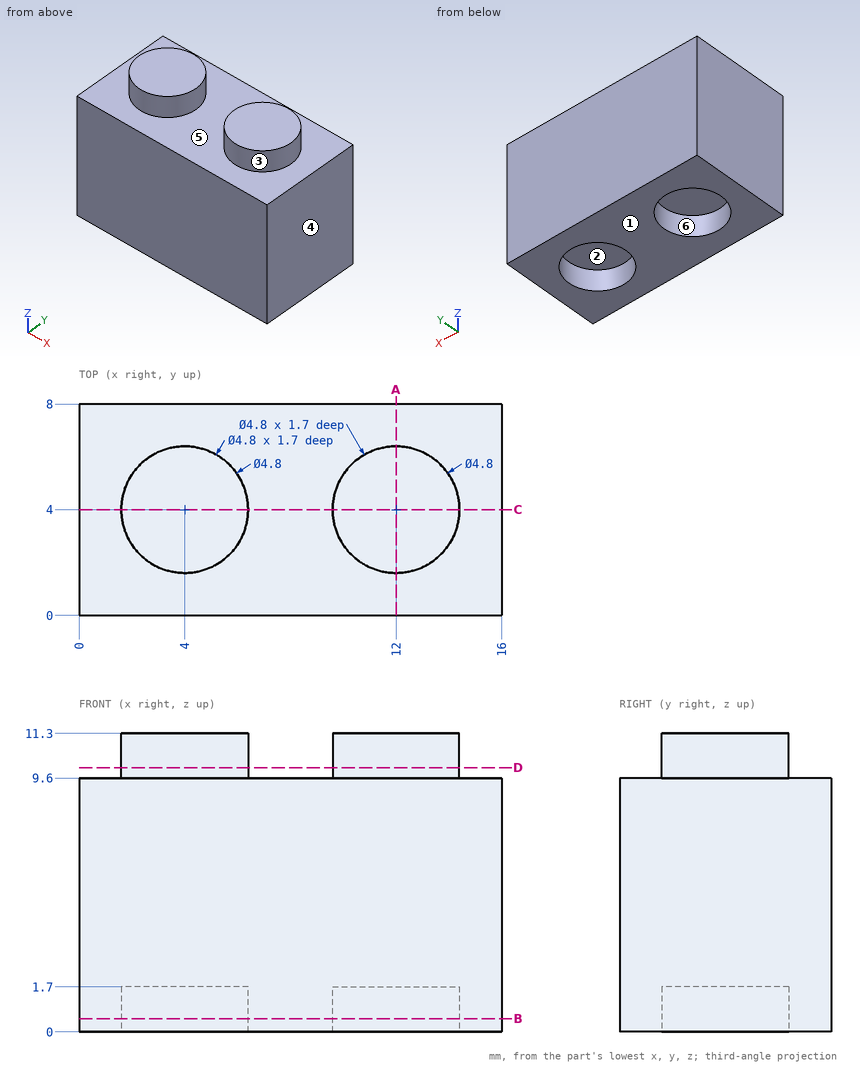
Could you check a few things on this drawing? It's one solid part, dimensions in mm from its lowest x, y, z. A direction names the side the tool comes from. Give positions to 0.01 mm unless a question says otherwise; leave off trailing zeros. Order: outer loops, then holes, each group sorted by start corner. A loop starts at its lowest first (then second) coordinate and runs counter-clockwise, first axis right, second up. Notation, with made-up numbers: (-39.75, 69) - (-7.75, 69) arc R16 cw to (-7.75, 74) - close; hole circle Ø2 at (76, 41). An arc over 180 degrees is marked (long way). Answer as a JSON object with one key per item and string values. Group by question number.
Item 1: Please list where these lines run through material, in increasing order: probe 1 along Y at (x, z) = (4, 0.8); probe 2 along X at (y, z) = (3.25, 1.25); probe 3 along Z at (x, y) = (8.25, 2).
Item 2: For P1, Ø4, axis at x = 12, y = 4.5, coming from the -Z side; P2, Ø2.5, axis at x = 3, y = 3.5, coming from the -Z side, each with a flat end and sliding along its axis, tell me the tip position at first contact or that it passes through.
Item 3: If we section it at D-D on z = 10: Please give me the cut outline in (x, y), and give its area (3 significant figures).
Item 4: If we section it at A-A on x = 12: Please give me the cut outline in (y, z), and give its area (3 significant figures).
Item 5: If we section it at C-C on y = 4: Please give me the cut outline in (x, z), and give its area (3 significant figures).
Item 6: If we section it at B-B on z = 0.5: Please give me the cut outline in (x, y), and give its area (3 significant figures).
Item 7: Which directions (+Z, -Z, +X, -X, +Y, -Y) give clear straight access to the entire face, cutting with the end or side of a thin tool? Please do the marked faces 4, 5 and 6.
Item 8: If we mould it in two halves opening along Y, with no side actions, what happens to the marked faces 1, 2 and 3? For each: pulls with the +Y half, pulls with the -Y half, needs draft (parallel to the pull), parting line crosses it, or undercut.
Result set:
{
 "1": {"probe 1": "0 to 1.6, 6.4 to 8", "probe 2": "0 to 1.72, 6.28 to 9.72, 14.28 to 16", "probe 3": "0 to 9.6"},
 "2": {"P1": "z = 0", "P2": "z = 1.7"},
 "3": {"outline": "circle Ø4.8 at (4, 4); circle Ø4.8 at (12, 4)", "area": "36.2 mm²"},
 "4": {"outline": "(0, 0) - (1.6, 0) - (1.6, 1.7) - (6.4, 1.7) - (6.4, 0) - (8, 0) - (8, 9.6) - (6.4, 9.6) - (6.4, 11.3) - (1.6, 11.3) - (1.6, 9.6) - (0, 9.6) - close", "area": "76.8 mm²"},
 "5": {"outline": "(0, 0) - (1.6, 0) - (1.6, 1.7) - (6.4, 1.7) - (6.4, 0) - (9.6, 0) - (9.6, 1.7) - (14.4, 1.7) - (14.4, 0) - (16, 0) - (16, 9.6) - (14.4, 9.6) - (14.4, 11.3) - (9.6, 11.3) - (9.6, 9.6) - (6.4, 9.6) - (6.4, 11.3) - (1.6, 11.3) - (1.6, 9.6) - (0, 9.6) - close", "area": "154 mm²"},
 "6": {"outline": "(0, 0) - (16, 0) - (16, 8) - (0, 8) - close; hole circle Ø4.8 at (4, 4); hole circle Ø4.8 at (12, 4)", "area": "91.8 mm²"},
 "7": {"face 4": "+Z, -Z, +X, +Y, -Y", "face 5": "+Z", "face 6": "-Z"},
 "8": {"face 1": "needs draft", "face 2": "undercut", "face 3": "parting line crosses it"}
}
